```python
from build123d import *

# Parameters (mm, degrees)
SKETCH1_W           = 55.8
SKETCH1_H           = 15.8
BOSS_EXTRUDE1_DEPTH = 28.8
SKETCH2_R           = 7.62
CUT_EXTRUDE1_DEPTH  = 12.7
SKETCH4_R           = 2.778125
SKETCH4_R_2         = 1.8415
CUT_EXTRUDE2_DEPTH  = 12.7
CUT_EXTRUDE6_DEPTH  = 1.905


with BuildPart() as part:
    # Sketch1 → Boss-Extrude1 (new body)
    with BuildSketch(Plane(origin=(0, 0, 0), x_dir=(1, 0, 0), z_dir=(0, 1, 0))):
        with Locations((-11.199948696, 8.193463303)):
            Rectangle(SKETCH1_W, SKETCH1_H)
    extrude(amount=BOSS_EXTRUDE1_DEPTH)

    # Sketch2 → Cut-Extrude1 (cut)
    with BuildSketch(Plane.XY.offset(-0.293463303)):
        with Locations((0.800051304, 15.4)):
            Circle(SKETCH2_R)
        with BuildLine():
            Line((-11.899948696, 10.6375), (-24.599948696, 10.6375))
            ThreePointArc((-24.599948696, 10.6375), (-29.362448696, 15.4), (-24.599948696, 20.1625))
            Line((-24.599948696, 20.1625), (-11.899948696, 20.1625))
            ThreePointArc((-11.899948696, 20.1625), (-7.137448696, 15.4), (-11.899948696, 10.6375))
        make_face()
    extrude(amount=-CUT_EXTRUDE1_DEPTH, mode=Mode.SUBTRACT)

    # Sketch4 → Cut-Extrude2 (cut)
    with BuildSketch(Plane(origin=(0, 0, -16.093463303), x_dir=(-1, 0, 0), z_dir=(0, 0, -1))):
        with Locations((-0.800051304, 15.4)):
            Circle(SKETCH4_R)
        with Locations((11.899948696, 15.4)):
            Circle(SKETCH4_R_2)
        with Locations((24.599948696, 15.4)):
            Circle(SKETCH4_R_2)
    extrude(amount=-CUT_EXTRUDE2_DEPTH, mode=Mode.SUBTRACT)

    # Sketch5 → Cut-Extrude6 (cut)
    with BuildSketch(Plane(origin=(0, 0, -16.093463303), x_dir=(-1, 0, 0), z_dir=(0, 0, -1))):
        with BuildLine():
            Line((24.599948696, 20.1625), (11.899948696, 20.1625))
            ThreePointArc((11.899948696, 20.1625), (7.137448696, 15.4), (11.899948696, 10.6375))
            Line((11.899948696, 10.6375), (24.599948696, 10.6375))
            ThreePointArc((24.599948696, 10.6375), (29.362448696, 15.4), (24.599948696, 20.1625))
        make_face()
    extrude(amount=-CUT_EXTRUDE6_DEPTH, mode=Mode.SUBTRACT)


solid = part.part
```
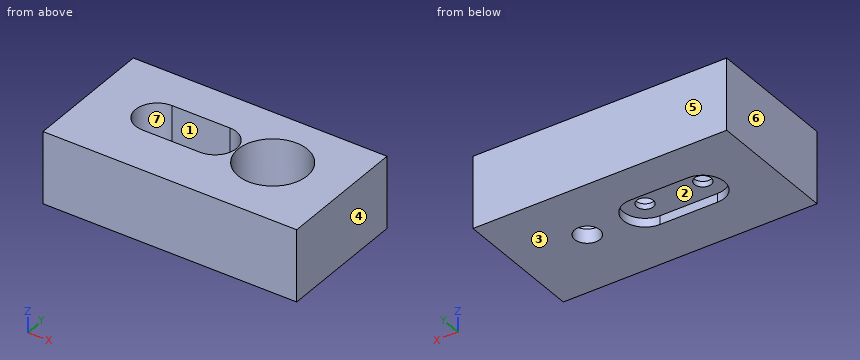
CAD build for the part. Positions are in the model's coordinates, mm. Face numbers are marked on the shaded views. A direction names the side the tool comes from. Round coordinates to 2 decimals unless told otherwise and drop trailing zeros. Order: outer loops, then holes, each group sorted by start corner. A loop starts at its lowest first (then second) coordinate and runs counter-clockwise, first axis right, second up. Notation, with made-up numbers: (87.25, 38.25) - (116.25, 38.25) arc R22 cw to (116.25, 47.25) - close; hole circle Ø5 at (-16, 70). An arc over 180 degrees is marked (long way). Answer in a Markdown table with one row per item. Add a question column.
(1) Probe L1, parallel to X at y = 13, z = -1.5; L2, parallel to X at y = 18.5, z = -2.25; L3, parallel to Y at x = -19.5, z = -2. List the from-to ranges inside material, lowest first. Write a range as [from, to].
(2) Band-saw the part on D-D on y = 11.25. List the corners of the cut face in (x, z).
(3) Band-saw the part on A-A on y = 15.4. List the corners of the cut face in (x, z), and give its area (3 significant figures).
(4) Band-saw the part on C-C on x = -21. List the corners of the cut face in (y, z), and give its area (3 significant figures).
(5) 3-axis set-ups, long thin cutter, end or side, ignore diameter. For the marked faces 1, 2 and 3: which of +Z, -Z, +X, -X, +Y, -Y reach the whole face in a straight line?
(6) Band-saw the part on B-B on z = -1.25. List the corners of the cut face in (x, y) (1 decimal).
(7) Mould opens along X. For the marked faces 4, 5, 6 and 7 say: +X half, -X half, draft (parallel to the pull), parting line (faces both ways), or undercut.
(8) Drop flat-ended pins along their axis: pin 1 Ø3 at (x, y) = (-19, 13.5) entering from -Z; pin 2 Ø6 at (x, y) = (-24.6, 15.4) entering from +Z. Give the stop position or say it passes through.
Data:
| question | item | result |
|---|---|---|
| 1 | L1 | x = [-39.1, -28.71], [-7.79, -6.43], [8.03, 16.7] |
| 1 | L2 | x = [-39.1, -28.22], [-8.28, -6.16], [7.76, 16.7] |
| 1 | L3 | y = [0, 10.64], [20.16, 28.8] |
| 2 | outline | (-39.1, -16.09) - (-26.94, -16.09) - (-26.94, -14.19) - (-9.56, -14.19) - (-9.56, -16.09) - (16.7, -16.09) - (16.7, -0.29) - (7.19, -0.29) - (7.19, -12.99) - (-5.59, -12.99) - (-5.59, -0.29) - (-9.56, -0.29) - (-9.56, -12.99) - (-26.94, -12.99) - (-26.94, -0.29) - (-39.1, -0.29) - close |
| 3 | outline | (-39.1, -16.09) - (-29.36, -16.09) - (-29.36, -14.19) - (-26.44, -14.19) - (-26.44, -12.99) - (-29.36, -12.99) - (-29.36, -0.29) - (-39.1, -0.29) - close; (-22.76, -14.19) - (-13.74, -14.19) - (-13.74, -12.99) - (-22.76, -12.99) - close; (-10.06, -14.19) - (-7.14, -14.19) - (-7.14, -16.09) - (-1.98, -16.09) - (-1.98, -12.99) - (-6.82, -12.99) - (-6.82, -0.29) - (-7.14, -0.29) - (-7.14, -12.99) - (-10.06, -12.99) - close; (3.58, -16.09) - (16.7, -16.09) - (16.7, -0.29) - (8.42, -0.29) - (8.42, -12.99) - (3.58, -12.99) - close |
| 3 | area | 337 mm^2 |
| 4 | outline | (0, -16.09) - (10.64, -16.09) - (10.64, -14.19) - (20.16, -14.19) - (20.16, -16.09) - (28.8, -16.09) - (28.8, -0.29) - (20.16, -0.29) - (20.16, -12.99) - (10.64, -12.99) - (10.64, -0.29) - (0, -0.29) - close |
| 4 | area | 316 mm^2 |
| 5 | face 1 | +Z |
| 5 | face 2 | -Z |
| 5 | face 3 | -Z, +X, -X, +Y, -Y |
| 6 | outline | (-39.1, 0) - (16.7, 0) - (16.7, 28.8) - (-39.1, 28.8) - close; hole (-24.6, 10.6) - (-11.9, 10.6) arc R4.8 ccw to (-11.9, 20.2) - (-24.6, 20.2) arc R4.8 ccw to start; hole circle Ø15.2 at (0.8, 15.4) |
| 7 | face 4 | +X half |
| 7 | face 5 | draft |
| 7 | face 6 | -X half |
| 7 | face 7 | undercut |
| 8 | pin 1 | stops at z = -14.19 |
| 8 | pin 2 | stops at z = -12.99 |
